```python
from build123d import *

# Parameters (mm, degrees)
F1_DEPTH     = 6
F2_R         = 2.5
F3_DEPTH     = 25
F4_T1_DEPTH  = 0.2
F4_T4_ANGLE  = 84.656067133
F4_T6_ANGLE  = 84.656067133
F4_T8_ANGLE  = 84.656067133
F4_T10_ANGLE = 84.656067133
F5_DEPTH     = 5


# Not quite as in the source:
# - a fillet or chamfer that OpenCascade refuses, or shapes differently, is made with other operations: its cross-section is extruded or revolved along the edge and cut away or added


with BuildPart() as f1:
    # F0 (on Top) → F1 (new body)
    with BuildSketch(Plane.XY):
        with BuildLine():
            Line((-3.071964772, 10.9479769804), (-3.271964772, 10.9479769804))
            ThreePointArc((-3.271964772, 10.9479769804), (-10.2723219058, 8.0483341141), (-13.171964772, 1.0479769804))
            Line((-13.171964772, 1.0479769804), (-13.171964772, 0.8479769804))
            ThreePointArc((-13.171964772, 0.8479769804), (-10.2723219058, -6.1523801534), (-3.271964772, -9.0520230196))
            Line((-3.271964772, -9.0520230196), (-3.071964772, -9.0520230196))
            ThreePointArc((-3.071964772, -9.0520230196), (3.9283923617, -6.1523801534), (6.828035228, 0.8479769804))
            Line((6.828035228, 0.8479769804), (6.828035228, 1.0479769804))
            ThreePointArc((6.828035228, 1.0479769804), (3.9283923617, 8.0483341141), (-3.071964772, 10.9479769804))
        make_face()
    extrude(amount=F1_DEPTH)

    # F2 (on face) → F3 (cut)
    with BuildSketch(Plane.XZ.offset(9.0520230196)):
        with Locations((-3.171964772, 5)):
            Circle(F2_R)
    extrude(amount=-F3_DEPTH, mode=Mode.SUBTRACT)

    # F4: chamfer of 0.5 on 2 edges, made by hand

    # F4_s2 → F4_t1 (cut)
    with BuildSketch(Plane.XZ.offset(-1.0479769804)):
        Polygon((-13.171964772, 5.5), (-12.671964772, 6), (-13.171964772, 6), align=None)
        Polygon((6.828035228, 5.5), (6.328035228, 6), (6.828035228, 6), align=None)
    extrude(amount=F4_T1_DEPTH, mode=Mode.SUBTRACT)

    # F4_s3 → F4_t4 (revolve, cut)
    with BuildSketch(Plane.XZ.offset(-1.0479769804)):
        Polygon((6.328035228, 6), (6.828035228, 5.5), (6.828035228, 6), align=None)
    revolve(axis=Axis((-3.071964772, 1.0479769804, 6), (0, 0, 1)), revolution_arc=F4_T4_ANGLE, mode=Mode.SUBTRACT)

    # F4_s5 → F4_t6 (revolve, cut)
    with BuildSketch(Plane(origin=(-3.1464057809, -0.2943167545, 0), x_dir=(0, 0, 1), z_dir=(0.9956535782, 0.0931340552, 0))):
        Polygon((5.5, -11.2481533781), (6, -10.7481533781), (6, -11.2481533781), align=None)
    revolve(axis=Axis((-3.271964772, 1.0479769804, 6), (0, 0, 1)), revolution_arc=F4_T6_ANGLE, mode=Mode.SUBTRACT)

    # F4_s7 → F4_t8 (revolve, cut)
    with BuildSketch(Plane.XZ.offset(-0.8479769804)):
        Polygon((-12.671964772, 6), (-13.171964772, 5.5), (-13.171964772, 6), align=None)
    revolve(axis=Axis((-3.271964772, 0.8479769804, 6), (0, 0, 1)), revolution_arc=F4_T8_ANGLE, mode=Mode.SUBTRACT)

    # F4_s9 → F4_t10 (revolve, cut)
    with BuildSketch(Plane(origin=(-2.9666864224, -0.2775056939, 0), x_dir=(0, 0, 1), z_dir=(-0.9956535782, -0.0931340552, 0))):
        Polygon((6, -8.2696041486), (5.5, -8.7696041486), (6, -8.7696041486), align=None)
    revolve(axis=Axis((-3.071964772, 0.8479769804, 6), (0, 0, 1)), revolution_arc=F4_T10_ANGLE, mode=Mode.SUBTRACT)

    # F5 (add): a face of the model
    f5_faces = [f1.faces().sort_by_distance(p)[0] for p in [
        (-3.171964772, 0.9479769804, 0),
    ]]
    extrude(f5_faces, amount=F5_DEPTH)


solid = f1.part
```
The model under review builds one solid part; all positions refer to its coordinate system, in mm. Round coordinates to 2 decimals unless told otherwise and drop trailing zeros. Order: outer loops, then holes, each group sorted by start corner. A loop starts at its lowest first (then second) coordinate and runs counter-clockwise, first axis right, second up. Notation, with made-up numbers: (23.25, 59.25) -> (61.25, 59.25) arc R26 cw to (61.25, 84.25) -> close; hole circle Ø8 at (-2, 11). An arc over 180 degrees is marked (long way). Use a Markdown table: item, result.
Q1. We need section B-B on z = -2.5. Write out the cut boundary in (x, y), then the cut area to 3 significant figures.
Values:
| item | result |
|---|---|
| outline | (-13.17, 0.85) arc R9.9 ccw to (-3.27, -9.05) -> (-3.07, -9.05) arc R9.9 ccw to (6.83, 0.85) -> (6.83, 1.05) arc R9.9 ccw to (-3.07, 10.95) -> (-3.27, 10.95) arc R9.9 ccw to (-13.17, 1.05) -> close |
| area | 316 mm^2 |
Q2. We need section D-D on x = -2.5. Write out the cut boundary in (y, z), then the cut area to 3 significant figures.
Values:
| item | result |
|---|---|
| outline | (-9.04, -5) -> (10.93, -5) -> (10.93, 2.59) -> (-9.04, 2.59) -> close |
| area | 152 mm^2 |
Q3. We need section C-C on z = 5. Write out the cut boundary in (x, y), then the cut area to 3 significant figures.
Values:
| item | result |
|---|---|
| outline | (-13.17, 0.85) arc R9.9 ccw to (-5.67, -8.76) -> (-5.67, 10.65) arc R9.9 ccw to (-13.17, 1.05) -> close; (-0.67, -8.76) arc R9.9 ccw to (6.83, 0.85) -> (6.83, 1.05) arc R9.9 ccw to (-0.67, 10.65) -> close |
| area | 217 mm^2 |
Q4. Clearance check with flat-ended pins moving along their axes: P1, Ø2, axis at x = 1, z = 4, coming from the -Y side; P2, Ø4, axis at x = -3.17, z = 5, coming from the +Y side; P3, Ø3, axis at y = -2.5, z = -3.5, coming from the +X side. State where each tip first meets the part, or that it passes through.
Values:
| item | result |
|---|---|
| P1 | stops at y = -8.56 |
| P2 | passes through |
| P3 | stops at x = 6.65 |
Q5. We need section A-A on z = 3. Write out the cut boundary in (x, y).
Values:
| item | result |
|---|---|
| outline | (-13.17, 0.85) arc R9.9 ccw to (-4.67, -8.95) -> (-4.67, 10.85) arc R9.9 ccw to (-13.17, 1.05) -> close; (-1.67, -8.95) arc R9.9 ccw to (6.83, 0.85) -> (6.83, 1.05) arc R9.9 ccw to (-1.67, 10.85) -> close |
Q6. For line 1 (X direction, y = -2.25, z = 5); line 2 (Y direction, x = -3.5, z = 0.5); line 3 (X direction, y = 2.75, z = 5), list the stretches that pass through material, from the lowest coordinate up.
Values:
| item | result |
|---|---|
| line 1 | x = -12.67 to -5.67, -0.67 to 6.33 |
| line 2 | y = -9.05 to 10.95 |
| line 3 | x = -13.02 to -5.67, -0.67 to 6.68 |
